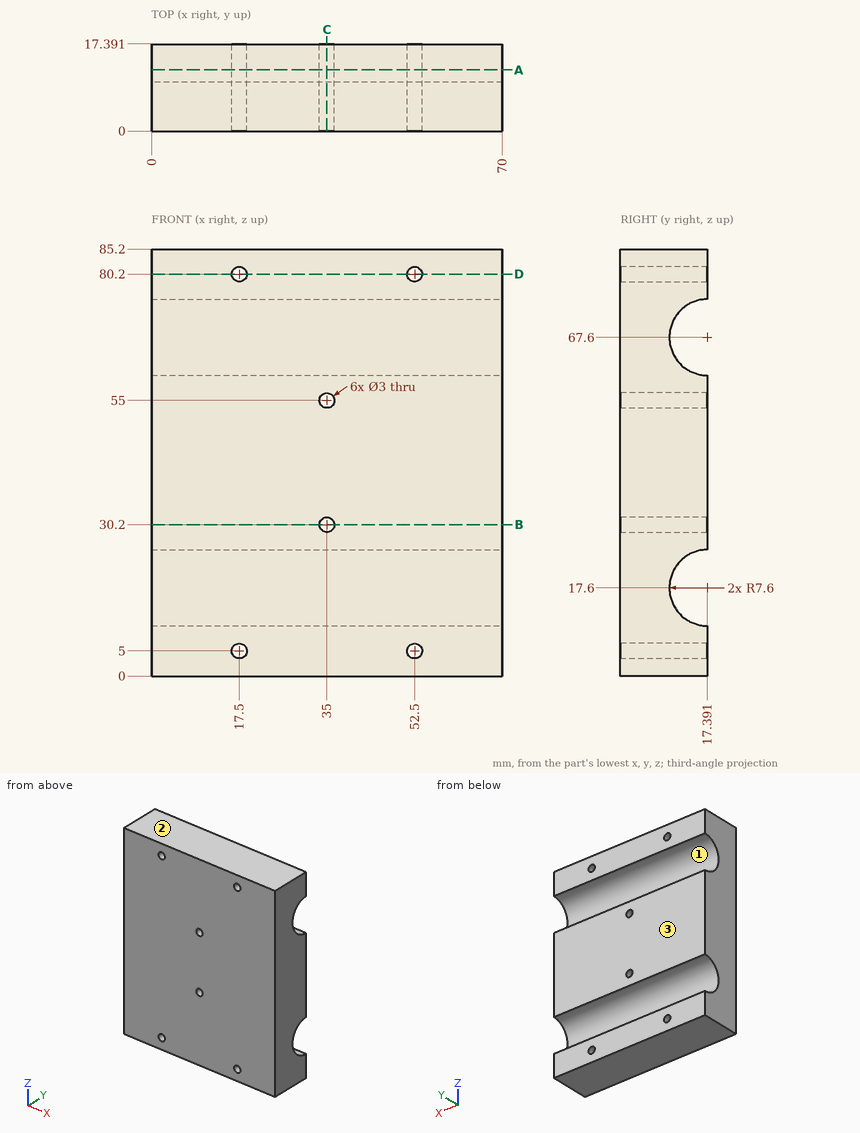
Job drawing, mm, ordinate dimensions from the low corner. One solid piece. Give positions to 0.01 mm unless a question says otherwise; leave off trailing zeros. Order: outer loops, then holes, each group sorted by start corner. A loop starts at its lowest first (then second) coordinate and runs counter-clockwise, first axis right, second up. Notation, with made-up numbers: M 40,-8.75 L 75,-8.75 A31 cw 75,25.25 Z; hole C 8,-7 d10. An arc over 180 degrees is marked long. Put each result on its own line as item: value. Start each with the question number.
(1) Band-saw the part on A-A on y = 12.25. Count the separate pieces of the cut face and the enclosed holes in it, then the cut area to 3 significant figures.
(2) Band-saw the part on D-D on z = 80.2. Give the cut face in (x, y).
(3) Pin check, flat tips, straight feed: pin 1 Ø1.8 at (x, z) = (52.5, 5) entering from -Y; pin 2 Ø1 at (x, z) = (33, 65) entering from +Y; pin 3 Ø10 at (x, z) = (56.5, 16) entering from +Y. Stop position of each tip, or through.
(4) Band-saw the part on C-C on x = 35. Give the cut face in (y, z), then the cut area to 3 significant figures.
(5) Drill centre lines: L1, parallel to X at y = 6.75, z = 80.2; L2, parallel to X at y = 7, z = 55; L3, parallel to Z at x = 43, y = 14. Where is each one in solid material? Low to high. Write a range as [from, to].
(6) Band-saw the part on B-B on z = 30.2. Give the cut face in (x, y).
(7) Pull direction Z, two halves, no side cores. Call the marked faces 1, 2 and 3: released by +Z, released by -Z, zero draft, split by the parting line, or undercut.
Results below:
1. separate pieces: 3
1. enclosed holes: 6
1. area: 4,350 mm2
2. outline: M 0,0 L 16,0 L 16,17.39 L 0,17.39 Z; M 19,0 L 51,0 L 51,17.39 L 19,17.39 Z; M 54,0 L 70,0 L 70,17.39 L 54,17.39 Z
3. pin 1: passes through
3. pin 2: stops at y = 10.45
3. pin 3: stops at y = 13.62
4. outline: M 0,0 L 17.39,0 L 17.39,10 A7.6 cw 17.39,25.2 L 17.39,28.7 L 0,28.7 Z; M 0,31.7 L 17.39,31.7 L 17.39,53.5 L 0,53.5 Z; M 0,56.5 L 17.39,56.5 L 17.39,60 A7.6 cw 17.39,75.2 L 17.39,85.2 L 0,85.2 Z
4. area: 1,200 mm2
5. L1: x = [0, 16], [19, 51], [54, 70]
5. L2: x = [0, 33.5], [36.5, 70]
5. L3: z = [0, 10.8], [24.4, 60.8], [74.4, 85.2]
6. outline: M 0,0 L 33.5,0 L 33.5,17.39 L 0,17.39 Z; M 36.5,0 L 70,0 L 70,17.39 L 36.5,17.39 Z
7. face 1: undercut
7. face 2: released by +Z
7. face 3: zero draft
